Design review of the part built by this model. Coordinates are the model's own, in mm. Give positions to 0.01 mm unless a question says otherwise; leave off trailing zeros. Answer as a JSON object with one key per item and string values.
```python
from build123d import *

# Parameters (mm, degrees)
SKETCH1_R           = 1.6
BOSS_EXTRUDE1_DEPTH = 0.8
CUT_EXTRUDE1_DEPTH  = 0.8


with BuildPart() as part:
    # Sketch1 → Boss-Extrude1 (new body)
    with BuildSketch(Plane.XY):
        Polygon((22.775267328, 35.726963173), (-59.324732672, 35.726963173), (-59.324732672, 29.126963173), (-67.024732672, 29.126963173), (-67.024732672, -9.073036827), (-62.524732672, -9.073036827), (-62.524732672, -15.073036827), (-67.024732672, -15.073036827), (-67.024732672, -53.173036827), (-59.424732672, -53.173036827), (-59.424732672, -60.773036827), (22.575267328, -60.773036827), (22.575267328, -53.173036827), (29.475267328, -53.173036827), (29.475267328, -15.073036827), (24.975267328, -15.073036827), (24.975267328, -9.073036827), (29.475267328, -9.073036827), (29.475267328, 29.126963173), (22.775267328, 29.126963173), align=None)
        with Locations((-18.724732672, -47.273036827)):
            Circle(SKETCH1_R, mode=Mode.SUBTRACT)
        with Locations((-54.124732672, -12.273036827)):
            Circle(SKETCH1_R, mode=Mode.SUBTRACT)
        with Locations((-5.624732672, 1.126963173)):
            Circle(SKETCH1_R, mode=Mode.SUBTRACT)
        with Locations((16.375267328, -12.273036827)):
            Circle(SKETCH1_R, mode=Mode.SUBTRACT)
        with Locations((-18.724732672, 23.126963173)):
            Circle(SKETCH1_R, mode=Mode.SUBTRACT)
    extrude(amount=BOSS_EXTRUDE1_DEPTH)

    # Sketch2 → Cut-Extrude1 (cut)
    with BuildSketch(Plane.XY.offset(0.8)):
        Polygon((-7.931660886, -9.465246416), (-16.416942261, -0.979965042), (-18.169105872, -2.732128653), (-9.683824497, -11.217410027), align=None)
        Polygon((-5.032523083, -6.566108613), (-13.517804458, 1.919172761), (-16.416942261, -0.979965042), (-7.931660886, -9.465246416), align=None)
        Polygon((-3.390574145, -4.924159675), (-11.875855519, 3.5611217), (-13.517804458, 1.919172761), (-5.032523083, -6.566108613), align=None)
    extrude(amount=-CUT_EXTRUDE1_DEPTH, mode=Mode.SUBTRACT)


solid = part.part
```
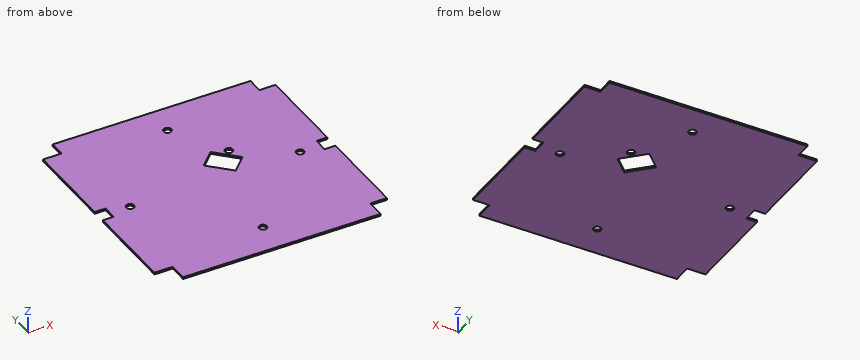
(1) For line 1 along X through (y, z) = (-12, 0.15); line 2 along Y through (x, z) = (25.5, 0.75); line 3 along X through (y, z) = (30, 0.75), list the stretches that pass through material, from the lowest coordinate up.
Here are the results:
{"line 1": "x = -62.52 to -55.7, -52.55 to 14.8, 17.95 to 24.98", "line 2": "y = -53.17 to -15.07, -9.07 to 29.13", "line 3": "x = -59.32 to 22.78"}
(2) We need section A-A, the plane z = 0.6. Give the number of separate pieces and of enclosed holes in the cut face, then the cut area to 3 significant figures.
Here are the results:
{"separate pieces": "1", "enclosed holes": "6", "area": "8,910 mm²"}
(3) Clearance check with a flat-ended pin moving along its axis: pin 1 (8 mm diameter, centred on x = 15, y = -10, fed in from -Z). State where the tip first meets the part, or that it passes through.
Here are the results:
{"pin 1": "stops at z = 0"}
